Part print with two shaded views. Sizes in mm from the minimum x, y, z corner. A direction names the side the tool comes from. Coordinates: 2 decimals unless noted, no trailing zeros. Loops run counter-clockwise (first coordinate to the right, second up) from the corner with the lowest first, then second, coordinate; pieces in that order, holes last.
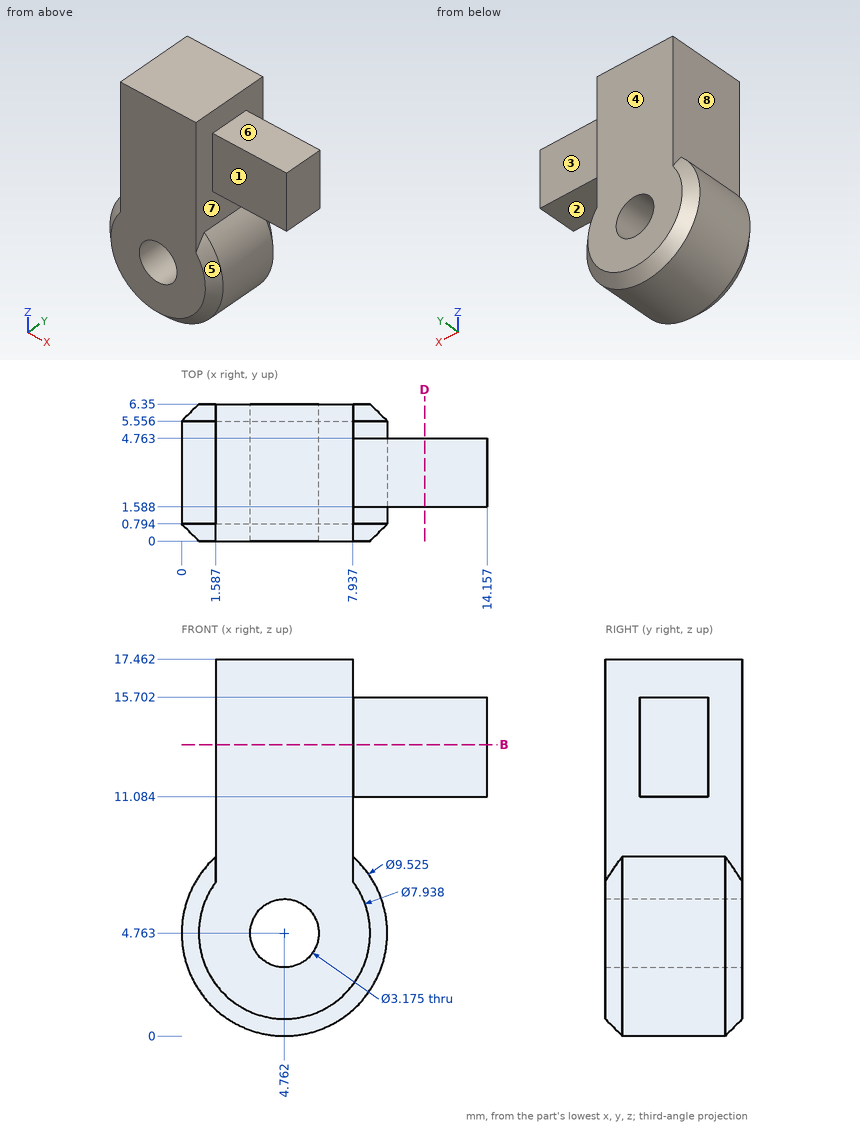
Q1. Mould opens along Z. For the marked faces 5, 6, 7 and 8 say: +Z half, -Z half, draft (parallel to the pull), parting line (faces both ways), or undercut.
Answers:
face 5: parting line
face 6: +Z half
face 7: undercut
face 8: draft
Q2. Slice it at B-B (z = 13.5). List the corners of the cut face in (x, y).
Answers:
outline: (1.59, 0) - (7.94, 0) - (7.94, 1.59) - (14.16, 1.59) - (14.16, 4.76) - (7.94, 4.76) - (7.94, 6.35) - (1.59, 6.35) - close
Q3. Drill centre lines: line 1 (X direction, y = 4, z = 11.5); line 2 (X direction, y = 0.5, z = 10); line 3 (Z direction, x = 3.5, y = 1.75) (1 decimal). Where is each one in solid material? Low to high.
Answers:
line 1: x = 1.59 to 14.16
line 2: x = 1.59 to 7.94
line 3: z = 0.2 to 3.8, 5.7 to 17.5
Q4. Slice it at D-D (x = 11.25). List the corners of the cut face in (y, z) (1 decimal).
Answers:
outline: (1.6, 11.1) - (4.8, 11.1) - (4.8, 15.7) - (1.6, 15.7) - close
Q5. Flat gauge pins, fed straight in: P1, Ø5, axis at x = 12, z = 12.5, coming from the +Y side; P2, Ø3.5, axis at x = 9.5, z = 12.5, coming from the -Y side; P3, Ø2.5, axis at x = 11, y = 2.5, coming from the +Z side; P4, Ø2.5, axis at x = 11, y = 3, coming from the -Z side. Where does each tip first touch, or does it go through?
Answers:
P1: stops at y = 4.76
P2: stops at y = 0
P3: stops at z = 15.7
P4: stops at z = 11.08
Q6. Which spindle directions (+Z, -Z, +X, -X, +Y, -Y) get a long thin tool onto all of the face, cutting with end or side? Do the marked faces 1, 2, 3 and 4. Say none if no direction does.
Answers:
face 1: +Z, +X, -Y
face 2: +X, +Y, -Y
face 3: +Z, +X, +Y
face 4: +Z, -Z, +X, -X, +Y
